```python
from build123d import *

# Parameters (mm, degrees)
CROQUIS1_W              = 3
CROQUIS1_H              = 3
SALIENTE_EXTRUIR1_DEPTH = 3


with BuildPart() as part:
    # Croquis1 → Saliente-Extruir1 (new body)
    with BuildSketch(Plane.XY):
        with BuildLine():
            Line((-30, -11.425), (-30, -8.425))
            Line((-30, -8.425), (-1.5, -8.425))
            Line((-1.5, -8.425), (-1.5, 30))
            Line((-1.5, 30), (-1.5, 33))
            Line((-1.5, 33), (-13, 33))
            ThreePointArc((-13, 33), (-27.142135624, 27.142135624), (-33, 13))
            Line((-33, 13), (-33, -13))
            ThreePointArc((-33, -13), (-31.515630385, -20.561179235), (-27.282856857, -27))
            Line((-27.282856857, -27), (-4.502856857, -27))
            Line((-4.502856857, -27), (-4.502856857, -30))
            Line((-4.502856857, -30), (-23.535653753, -30))
            ThreePointArc((-23.535653753, -30), (-18.477225575, -32.235384062), (-13, -33))
            Line((-13, -33), (13, -33))
            ThreePointArc((13, -33), (18.477225575, -32.235384062), (23.535653753, -30))
            Line((23.535653753, -30), (4.502856857, -30))
            Line((4.502856857, -30), (4.502856857, -27))
            Line((4.502856857, -27), (27.282856857, -27))
            ThreePointArc((27.282856857, -27), (31.515630385, -20.561179235), (33, -13))
            Line((33, -13), (33, 13))
            ThreePointArc((33, 13), (27.142135624, 27.142135624), (13, 33))
            Line((13, 33), (1.5, 33))
            Line((1.5, 33), (1.5, 30))
            Line((1.5, 30), (1.5, -8.425))
            Line((1.5, -8.425), (30, -8.425))
            Line((30, -8.425), (30, -11.425))
            Line((30, -11.425), (1.5, -11.425))
            Line((1.5, -11.425), (1.5, -30))
            Line((1.5, -30), (-1.5, -30))
            Line((-1.5, -30), (-1.5, -11.425))
            Line((-1.5, -11.425), (-30, -11.425))
        make_face()
        with Locations((-23.5, -16.1)):
            Rectangle(CROQUIS1_W, CROQUIS1_H, mode=Mode.SUBTRACT)
        with Locations((-12.5, -16.1)):
            Rectangle(CROQUIS1_W, CROQUIS1_H, mode=Mode.SUBTRACT)
        with Locations((12.5, -16.1)):
            Rectangle(CROQUIS1_W, CROQUIS1_H, mode=Mode.SUBTRACT)
        with Locations((23.5, -16.1)):
            Rectangle(CROQUIS1_W, CROQUIS1_H, mode=Mode.SUBTRACT)
        with Locations((-5.5, 16.4)):
            Rectangle(CROQUIS1_W, CROQUIS1_H, mode=Mode.SUBTRACT)
        with Locations((5.5, 16.4)):
            Rectangle(CROQUIS1_W, CROQUIS1_H, mode=Mode.SUBTRACT)
    extrude(amount=SALIENTE_EXTRUIR1_DEPTH)


solid = part.part
```
The listing builds one solid part. Answer for the finished solid, in the listing's coordinates (mm). A direction names the side the tool comes from. Give positions to 0.01 mm unless a question says otherwise; leave off trailing zeros. Write each loop counter-clockwise with the first axis right and the second up, starting at its lowest first coordinate (ties: lowest second). Pieces come first, ordered by that corner, then holes. Notation, with made-up numbers: (-3.5, -27) -> (2.5, -27) arc R19 ccw to (2.5, -7) -> close; hole circle Ø6 at (88.5, 69.25). An arc over 180 degrees is marked (long way). Use one line per item in the form item = value.
1) Each of these flat-tipped pins is pushed along its axis until it touches: P1, Ø6, axis at x = -13.5, y = -11.5, coming from the -Z side; P2, Ø1.5, axis at x = -15.5, z = 2, coming from the +Y side; P3, Ø0.9, axis at y = -16, z = 1, coming from the +X side; P4, Ø0.9, axis at y = -29, z = 1, coming from the +X side. Where does it stop, or does it pass through?
Result:
P1 = 0
P2 = 32.92
P3 = 32.84
P4 = 4.5
2) A tool of negligible diameter and unlimited length cuts with its end or side. For faces 4 (the flat face through (-6, 14.9, 1)), 5 (the cylindrical face through (27.297, 26.986, 1.479)), 6 (the flat face through (-8, 0, 3)), 7 (the flat face through (-4.503, -28, 1)), 8 (the flat face through (-1.5, -21, 1)), from which of +Z, -Z, +X, -X, +Y, -Y can it reach the whole face along a straight path? Write none if from no direction.
Result:
face_4 = +Z, -Z
face_5 = +Z, -Z, +X, +Y
face_6 = +Z, +X, -X, +Y, -Y
face_7 = +Z, -Z, -X
face_8 = +Z, -Z, +Y
3) Section B-B on x = -21 is taken. Write down the section's boundary in (y, z) (3 decimals), plus the area to 3 significant figures.
Result:
outline = (-31.33, 0) -> (-30, 0) -> (-30, 3) -> (-31.33, 3) -> close; (-27, 0) -> (-11.425, 0) -> (-11.425, 3) -> (-27, 3) -> close; (-8.425, 0) -> (31.33, 0) -> (31.33, 3) -> (-8.425, 3) -> close
area = 170 mm²
4) Section A-A on x = 6 is taken. Write down the section's boundary in (y, z) (3 decimals), plus the area to 3 significant figures.
Result:
outline = (-33, 0) -> (-30, 0) -> (-30, 3) -> (-33, 3) -> close; (-27, 0) -> (-11.425, 0) -> (-11.425, 3) -> (-27, 3) -> close; (-8.425, 0) -> (14.9, 0) -> (14.9, 3) -> (-8.425, 3) -> close; (17.9, 0) -> (33, 0) -> (33, 3) -> (17.9, 3) -> close
area = 171 mm²
5) Straight lines are drawn through the part: probe 1 along Y at (x, z) = (-5.5, 2.55) (3 decimals); probe 2 along Y at (x, z) = (9, 0.3) (3 decimals); probe 3 along X at (y, z) = (1, 1.15). For each, find the intervals that lie inside material, in ascending order.
Result:
probe_1 = -33 to -30, -27 to -11.425, -8.425 to 14.9, 17.9 to 33
probe_2 = -33 to -30, -27 to -11.425, -8.425 to 33
probe_3 = -33 to -1.5, 1.5 to 33
6) Section C-C on y = 25.5 is taken. Write down the section's boundary in (x, z), plus the area to 3 significant figures.
Result:
outline = (-28.61, 0) -> (-1.5, 0) -> (-1.5, 3) -> (-28.61, 3) -> close; (1.5, 0) -> (28.61, 0) -> (28.61, 3) -> (1.5, 3) -> close
area = 163 mm²
7) For a pull along Y with two mould halves and no side action, classify faces 1 (the cylindrical face through (-18.6, -32.2, 1.5)), 2 (the flat face through (7, 33, 1)), 3 (the flat face through (30, -10, 1)) as +Y half, -Y half, draft (parallel to the pull), parting line (faces both ways), or undercut.
Result:
face_1 = -Y half
face_2 = +Y half
face_3 = undercut
8) Section D-D on z = 1.45 is taken. Count the separate pieces of the cut face and the enclosed holes in it, plus the area to 3 significant figures.
Result:
separate_pieces = 1
enclosed_holes = 6
area = 3,470 mm²
